Geometry: final body of the model. Coordinates: model frame, mm. A direction names the side the tool comes from. Give positions to 0.01 mm unless a question says otherwise; leave off trailing zeros. Loops run counter-clockwise (first coordinate to the right, second up) from the corner with the lowest first, then second, coordinate; pieces in that order, holes last. Notation, with made-up numbers: (-3, 4.5) -> (13, 4.5) arc R15 cw to (13, 8.5) -> close; hole circle Ø1 at (23, -6). An arc over 180 degrees is marked (long way). One line per question, with ' | ' between items. Start each with the question number.
Item 1: Section C-C on x = 15.5. Return loops of the section in (y, z), then the cut area to 3 significant figures.
Item 2: Section D-D on y = 11.25. Return loops of the section in (x, z), then the cut area to 3 significant figures.
Item 3: Section B-B on z = 3.1. Return loops of the section in (x, y).
Item 4: Material intervals for line 1 along X through (y, z) = (16, 1.55); line 2 along X through (y, z) = (-0.75, 4.3); line 3 along Y through (x, z) = (46.5, 2.1), sorted ascending. Write a range as [from, to].
Item 5: Set-up query: faces 4 (the flat face through (40, 3.928, 2)), 5 (the flat face through (37, -3.928, 2)). Return all of +Z, -Z, +X, -X, +Y, -Y with unobstructed straight access to the full face (end or side cutting, diameter ignored); none if empty.
Item 6: Mould query, pull axis X, two halves, no side actions, for faces 1 (the flat face through (29, 2, 0)), 2 (the cylindrical face through (66.773, 0.451, 2.465)), 3 (the cylindrical face through (8.536, -3.391, 2.465)). Classes: released by +X, released by -X, zero draft, split by the parting line, or undercut.
Item 7: Pin query (flat end, axial travel): P1, Ø2, axis at y = 3.5, z = 2, coming from the -X side; P2, Ø2, axis at y = 7.5, z = 4, coming from the +X side; P3, Ø3, axis at y = 14, z = 1.5, coming from the +X side; P4, Ø2.5, axis at x = 65.34, y = 0, coming from the -Z side. Return the tip coordinate at first contact, or that it passes through.
Item 8: Section A-A on y = 0. Return loops of the section in (x, z).
from build123d import *

# Parameters (mm, degrees)
SKETCH1_R           = 1.5
BOSS_EXTRUDE2_DEPTH = 5


with BuildPart() as part:
    # Sketch1 → Boss-Extrude2 (new body)
    with BuildSketch(Plane.XY):
        with BuildLine():
            ThreePointArc((1.550594596, 18.168790447), (-4.235995189, 18.799274261), (-4.866479002, 13.012684476))
            Line((-4.866479002, 13.012684476), (7.66064778, -2.578052986))
            ThreePointArc((7.66064778, -2.578052986), (8.549937722, -3.400317574), (9.640055191, -3.928142886))
            Line((9.640055191, -3.928142886), (65.342057797, -3.928142886))
            ThreePointArc((65.342057797, -3.928142886), (69.270200683, 0), (65.342057797, 3.928142886))
            Line((65.342057797, 3.928142886), (48.461164636, 3.928142886))
            Line((48.461164636, 3.928142886), (12.992926807, 3.928142886))
            Line((12.992926807, 3.928142886), (4.83629607, 14.07954397))
            Line((4.83629607, 14.07954397), (1.550594596, 18.168790447))
        make_face()
        with Locations((-1.657942203, 15.590737462)):
            Circle(SKETCH1_R, mode=Mode.SUBTRACT)
        with Locations((65.342057797, 0)):
            Circle(SKETCH1_R, mode=Mode.SUBTRACT)
    extrude(amount=BOSS_EXTRUDE2_DEPTH)


solid = part.part
Result sheet:
1) outline: (-3.93, 0) -> (3.93, 0) -> (3.93, 5) -> (-3.93, 5) -> close | area: 39.3 mm²
2) outline: (-3.45, 0) -> (7.11, 0) -> (7.11, 5) -> (-3.45, 5) -> close | area: 52.8 mm²
3) outline: (-4.87, 13.01) -> (7.66, -2.58) arc R4.12 ccw to (9.64, -3.93) -> (65.34, -3.93) arc R3.93 ccw to (65.34, 3.93) -> (12.99, 3.93) -> (1.55, 18.17) arc R4.12 ccw to start; hole circle Ø3 at (-1.66, 15.59); hole circle Ø3 at (65.34, 0)
4) line 1: x = [-5.75, -3.1], [-0.21, 3.29] | line 2: x = [6.19, 64.04], [66.64, 69.2] | line 3: y = [-3.93, 3.93]
5) face 4: +Z, -Z, +X, +Y | face 5: +Z, -Z, +X, -X, -Y
6) face 1: zero draft | face 2: undercut | face 3: released by -X
7) P1: stops at x = 1.97 | P2: stops at x = 10.93 | P3: stops at x = 6.11 | P4: passes through
8) outline: (5.59, 0) -> (63.84, 0) -> (63.84, 5) -> (5.59, 5) -> close; (66.84, 0) -> (69.27, 0) -> (69.27, 5) -> (66.84, 5) -> close
